```python
from build123d import *

# Parameters (mm, degrees)
BOSS_EXTRUDE1_DEPTH = 3
SKETCH2_W           = 31.541335057
SKETCH2_H           = 3.08
CUT_EXTRUDE1_DEPTH  = 3


with BuildPart() as part:
    # Sketch1 → Boss-Extrude1 (new body)
    with BuildSketch(Plane.XY):
        with BuildLine():
            Line((12.452839565, 41.33272136), (-20, 4))
            Line((-20, 4), (-12, 4))
            Line((-12, 4), (-12, 0))
            Line((-12, 0), (12, 0))
            Line((12, 0), (12, 4))
            Line((12, 4), (20, 4))
            Line((20, 4), (42.354172484, 29.715533795))
            ThreePointArc((42.354172484, 29.715533795), (46.774384872, 33.016262939), (52.165397026, 34.186766418))
            Line((52.165397026, 34.186766418), (100.240955705, 34.186766418))
            ThreePointArc((100.240955705, 34.186766418), (100.86429233, 34.485317067), (101.02238507, 35.158137789))
            ThreePointArc((101.02238507, 35.158137789), (102.836349044, 51.235945442), (114.085991202, 62.864871253))
            ThreePointArc((114.085991202, 62.864871253), (114.498680148, 63.764494769), (113.721018225, 64.376766418))
            Line((113.721018225, 64.376766418), (63.01838144, 64.376766418))
            ThreePointArc((63.01838144, 64.376766418), (35.233934182, 58.344171567), (12.452839565, 41.33272136))
        make_face()
    extrude(amount=BOSS_EXTRUDE1_DEPTH)

    # Sketch2 → Cut-Extrude1 (cut)
    with BuildSketch(Plane.XY.offset(3)):
        with Locations((5.229332471, 30.5)):
            Rectangle(SKETCH2_W, SKETCH2_H)
    extrude(amount=-CUT_EXTRUDE1_DEPTH, mode=Mode.SUBTRACT)


solid = part.part
```
Check sheet for the modelled part. Datum: model origin and axes. Units: mm. A direction names the side the tool comes from. Coordinates: 2 decimals unless noted, no trailing zeros. Write each loop counter-clockwise with the first axis right and the second up, starting at its lowest first coordinate (ties: lowest second). Pieces come first, ordered by that corner, then holes. Notation, with made-up numbers: (70.5, 29.5) - (107.5, 29.5) arc R11 cw to (107.5, 38.5) - close; hole circle Ø6 at (-20.5, 72). An arc over 180 degrees is marked (long way). One line per question, with ' | ' between items.
Item 1: Access from +Z, -Z, +X, -X, +Y, -Y to the whole of each face (thin tool, end or side, straight path). Record for faces 4 (the face through (16, 4, 1)), 5 (the face through (-16, 4, 1)), 6 (the face through (13, 32.04, 2)).
Determined:
face 4: +Z, -Z, +X, -Y | face 5: +Z, -Z, -X, -Y | face 6: +Z, -Z, -X
Item 2: Gauge pin test, flat end, axial feed: P1, Ø1.5, axis at y = 20.5, z = 2.5, coming from the +X side. Record the tip position at first contact, or that the pin passes through.
Determined:
P1: stops at x = 35
Item 3: Thickness scan on line 1 (Y direction, x = 98, z = 2.4); line 2 (Y direction, x = 10.5, z = 0.1); line 3 (Y direction, x = 20, z = 1.2). Record the ranges inside material, lowest first. Write a range as [from, to].
Determined:
line 1: y = [34.19, 64.38] | line 2: y = [0, 28.96], [32.04, 39.09] | line 3: y = [4, 28.96], [32.04, 48.74]
Item 4: Sectioned sample at B-B on z = 1.8. Record the boundary of the cut face in (x, y), plus the area to 3 significant figures.
Determined:
outline: (-20, 4) - (-12, 4) - (-12, 0) - (12, 0) - (12, 4) - (20, 4) - (42.35, 29.72) arc R13 cw to (52.17, 34.19) - (100.24, 34.19) arc R0.8 ccw to (101.02, 35.16) arc R25.09 cw to (114.09, 62.86) arc R0.8 ccw to (113.72, 64.38) - (63.02, 64.38) arc R67 ccw to (12.45, 41.33) - (4.37, 32.04) - (21, 32.04) - (21, 28.96) - (1.7, 28.96) - close | area: 3,680 mm2
Item 5: Mould release check, pull along Y, two halves, no side actions. Record for faces 1 (the face through (46.7, 32.98, 1.48)), 2 (the face through (35.6, 58.51, 1.48)), 3 (the face through (21, 30, 2)): pulls with the +Y half, pulls with the -Y half, needs draft (parallel to the pull), parting line crosses it, or undercut.
Determined:
face 1: pulls with the -Y half | face 2: pulls with the +Y half | face 3: undercut
Item 6: Sectioned sample at A-A on x = 65. Record the boundary of the cut face in (y, z).
Determined:
outline: (34.19, 0) - (64.38, 0) - (64.38, 3) - (34.19, 3) - close
Item 7: Sectioned sample at C-C on y = 22.5. Record the boundary of the cut face in (x, z).
Determined:
outline: (-3.92, 0) - (36.08, 0) - (36.08, 3) - (-3.92, 3) - close
